```python
from build123d import *

# Parameters (mm, degrees)
SKETCH1_R                 = 5
BOSS_EXTRUDE1_DEPTH       = 58.42
F_4_40_TAPPED_HOLE1_D     = 2.2606
F_4_40_TAPPED_HOLE1_DEPTH = 9.525
F_4_40_TAPPED_HOLE1_TIP   = 0.679152758
F_4_40_TAPPED_HOLE2_D     = 2.2606
F_4_40_TAPPED_HOLE2_DEPTH = 9.525
F_4_40_TAPPED_HOLE2_TIP   = 0.679152758
SKETCH7_R                 = 0.635
CUT_EXTRUDE1_DEPTH        = 6
CUT_EXTRUDE1_DEPTH_BACK   = 6


with BuildPart() as part:
    # Sketch1 → Boss-Extrude1 (new body)
    with BuildSketch(Plane(origin=(0, 0, 0), x_dir=(1, 0, 0), z_dir=(0, 1, 0))):
        with Locations(Location((0, 0, 0), (0, 0, 270))):  # turned: the seam where the file's is
            Circle(SKETCH1_R)
    extrude(amount=BOSS_EXTRUDE1_DEPTH)

    # #4-40 Tapped Hole1
    with Locations(Plane(origin=(0, 58.42, 0), x_dir=(1, 0, 0), z_dir=(0, 1, 0))):
        with Locations((0, 0)):
            Hole(F_4_40_TAPPED_HOLE1_D / 2, depth=F_4_40_TAPPED_HOLE1_DEPTH)
            with Locations((0, 0, -(F_4_40_TAPPED_HOLE1_DEPTH + F_4_40_TAPPED_HOLE1_TIP / 2))):  # 118° drill point
                Cone(0, F_4_40_TAPPED_HOLE1_D / 2, F_4_40_TAPPED_HOLE1_TIP, mode=Mode.SUBTRACT)

    # #4-40 Tapped Hole2
    with Locations(Plane(origin=(0, 0, 0), x_dir=(-1, 0, 0), z_dir=(0, -1, 0))):
        with Locations((0, 0)):
            Hole(F_4_40_TAPPED_HOLE2_D / 2, depth=F_4_40_TAPPED_HOLE2_DEPTH)
            with Locations((0, 0, -(F_4_40_TAPPED_HOLE2_DEPTH + F_4_40_TAPPED_HOLE2_TIP / 2))):  # 118° drill point
                Cone(0, F_4_40_TAPPED_HOLE2_D / 2, F_4_40_TAPPED_HOLE2_TIP, mode=Mode.SUBTRACT)

    # Sketch7 → Cut-Extrude1 (cut, two sides)
    with BuildSketch(Plane.XY) as cut_extrude1_sk:
        with Locations((0, 49.657)):
            Circle(SKETCH7_R)
        with Locations((0, 8.763)):
            Circle(SKETCH7_R)
    extrude(amount=CUT_EXTRUDE1_DEPTH, mode=Mode.SUBTRACT)
    extrude(cut_extrude1_sk.sketch, amount=-CUT_EXTRUDE1_DEPTH_BACK, mode=Mode.SUBTRACT)


solid = part.part
```
Geometry check sheet. Reference: the model listing, model coordinates, mm. A direction names the side the tool comes from. Round coordinates to 2 decimals unless told otherwise and drop trailing zeros. Loops run counter-clockwise (first coordinate to the right, second up) from the corner with the lowest first, then second, coordinate; pieces in that order, holes last. Notation, with made-up numbers: (21.5, 37) - (34.5, 37) arc R19 cw to (34.5, 44) - close; hole circle Ø6 at (44, 41). An arc over 180 degrees is marked (long way). Use a Markdown table: item, result.
Q1. Cross-section at C-C on x = -1.75. Record the cut outline in (y, z), plus the area to 3 significant figures.
Solutions:
| item | result |
|---|---|
| outline | (0, -4.68) - (58.42, -4.68) - (58.42, 4.68) - (0, 4.68) - close |
| area | 547 mm2 |
Q2. Cross-section at A-A on z = -2. Record the cut outline in (x, y) (3 decimals).
Solutions:
| item | result |
|---|---|
| outline | (-4.583, 0) - (4.583, 0) - (4.583, 58.42) - (-4.583, 58.42) - close; hole circle Ø1.27 at (0, 8.763); hole circle Ø1.27 at (0, 49.657) |
Q3. Access from +Z, -Z, +X, -X, +Y, -Y to the whole of each face (thin tool, end or side, straight path). Record for faces 5 (the cylindrical face through (0.15, 53.59, -1.12)), 6 (the cylindrical face through (-0.15, 4.83, -1.12)), 7 (the cylindrical face through (-0.138, 8.143, 2.939)).
Solutions:
| item | result |
|---|---|
| face 5 | +Y |
| face 6 | -Y |
| face 7 | +Z, -Z |
Q4. Cross-section at B-B on y = 4.5. Record the cut outline in (x, z), plus the area to 3 significant figures.
Solutions:
| item | result |
|---|---|
| outline | circle Ø10 at (0, 0); hole circle Ø2.26 at (0, 0) |
| area | 74.5 mm2 |
Q5. Go/stop test with flat-tipped pins: P1, Ø1, axis at x = 0, y = 49.657, coming from the -Z side; P2, Ø1, axis at y = 28.5, z = -3, coming from the -X side; P3, Ø2, axis at x = 0, z = 0, coming from the +Y side; P4, Ø3, axis at x = 3.5, y = 20, coming from the +Z side. Record where each tip stops, or that it passes through.
Solutions:
| item | result |
|---|---|
| P1 | passes through |
| P2 | stops at x = -4.33 |
| P3 | stops at y = 48.82 |
| P4 | stops at z = 4.58 |
Q6. Material ranges on line 1 (Y direction, x = 0, z = -2.2); line 2 (Z direction, x = 0, y = 4.5); line 3 (Y direction, x = -0.25, z = -4.25), recorded low to high.
Solutions:
| item | result |
|---|---|
| line 1 | y = 0 to 8.13, 9.4 to 49.02, 50.29 to 58.42 |
| line 2 | z = -5 to -1.13, 1.13 to 5 |
| line 3 | y = 0 to 8.18, 9.35 to 49.07, 50.24 to 58.42 |
Q7. Draft check along Y on faces 1 (the cylindrical face through (1.5, 28.8, 4.77)), 2 (the cylindrical face through (-0.138, 8.143, -2.939)), 3 (the conical face through (0.043, 10.086, 0.192)), 4 (the conical face through (-0.156, 48.334, 0.119)). Enter one of: released by +Y, released by -Y, zero draft, split by the parting line, or undercut.
Solutions:
| item | result |
|---|---|
| face 1 | zero draft |
| face 2 | undercut |
| face 3 | released by -Y |
| face 4 | released by +Y |
Q8. Cross-section at D-D on y = 14. Record the cut outline in (x, z).
Solutions:
| item | result |
|---|---|
| outline | circle Ø10 at (0, 0) |
